from build123d import *

# Parameters (mm, degrees)
F1_DEPTH = 101.6
F2_W     = 19.05
F2_H     = 50.8
F3_DEPTH = 25.4


with BuildPart() as f1:
    # F0 (on Top) → F1 (new body)
    with BuildSketch(Plane.XY):
        Polygon((609.6, -9.525), (609.6, 0), (609.6, 9.525), (-609.6, 9.525), (-609.6, 0), (-609.6, -9.525), align=None)
    extrude(amount=-F1_DEPTH)

    # F2 (on face) → F3 (cut)
    with BuildSketch(Plane.XZ.offset(9.525)):
        with Locations((-396.875, -76.2)):
            Rectangle(F2_W, F2_H)
        with Locations((396.875, -76.2)):
            Rectangle(F2_W, F2_H)
    extrude(amount=-F3_DEPTH, mode=Mode.SUBTRACT)


solid = f1.part
Design review of the part built by this model. Coordinates are the model's own, in mm. A direction names the side the tool comes from. Round coordinates to 2 decimals unless told otherwise and drop trailing zeros. Loops run counter-clockwise (first coordinate to the right, second up) from the corner with the lowest first, then second, coordinate; pieces in that order, holes last. Notation, with made-up numbers: (-6, -3) -> (21, -3) arc R19 ccw to (21, 20) -> close; hole circle Ø2 at (34.25, -14). An arc over 180 degrees is marked (long way). Use one line per item in the form item = value. Start each with the question number.
Q1. For pin 1 Ø10 at (x, y) = (-132.5, 2.5) entering from +Z; pin 2 Ø9.5 at (x, y) = (-395, -3) entering from -Z, all flat-tipped, find the tip position at first contact; note any pin that passes through.
Q2. Draft analysis for pull direction X (two halves, no side actions). For faces 3 (the face through (609.6, 0, -50)), 4 (the face through (-5, 0, -101.6)), 5 (the face through (-387.35, 0, -77)), state which applies: +X half, -X half, draft (parallel to the pull), parting line (faces both ways), or undercut.
Q3. Machinability: for faces 1 (the face through (387.35, 0, -77)), 2 (the face through (9, 9.525, -50)), which of the approach directions +Z, -Z, +X, -X, +Y, -Y give a long, thin tool a straight path to every point of the face, cutting with its end or side? Answer none if there is none.
Q4. We need section A-A on y = 4. Give the boundary of the cut face in (x, z), then the cut area to 3 significant figures.
Q5. Wall thickness on line 1 along X through (y, z) = (-6, -81.5): over which ranges is the line inside the solid? List them lowest first. Write a range as [from, to].
Calculated:
q1.pin_1 = 0
q1.pin_2 = -50.8
q2.face_3 = +X half
q2.face_4 = draft
q2.face_5 = undercut
q3.face_1 = -Z, +Y, -Y
q3.face_2 = +Z, -Z, +X, -X, +Y
q4.outline = (-609.6, -101.6) -> (-406.4, -101.6) -> (-406.4, -50.8) -> (-387.35, -50.8) -> (-387.35, -101.6) -> (387.35, -101.6) -> (387.35, -50.8) -> (406.4, -50.8) -> (406.4, -101.6) -> (609.6, -101.6) -> (609.6, 0) -> (-609.6, 0) -> close
q4.area = 122,000 mm²
q5.line_1 = [-609.6, -406.4], [-387.35, 387.35], [406.4, 609.6]
